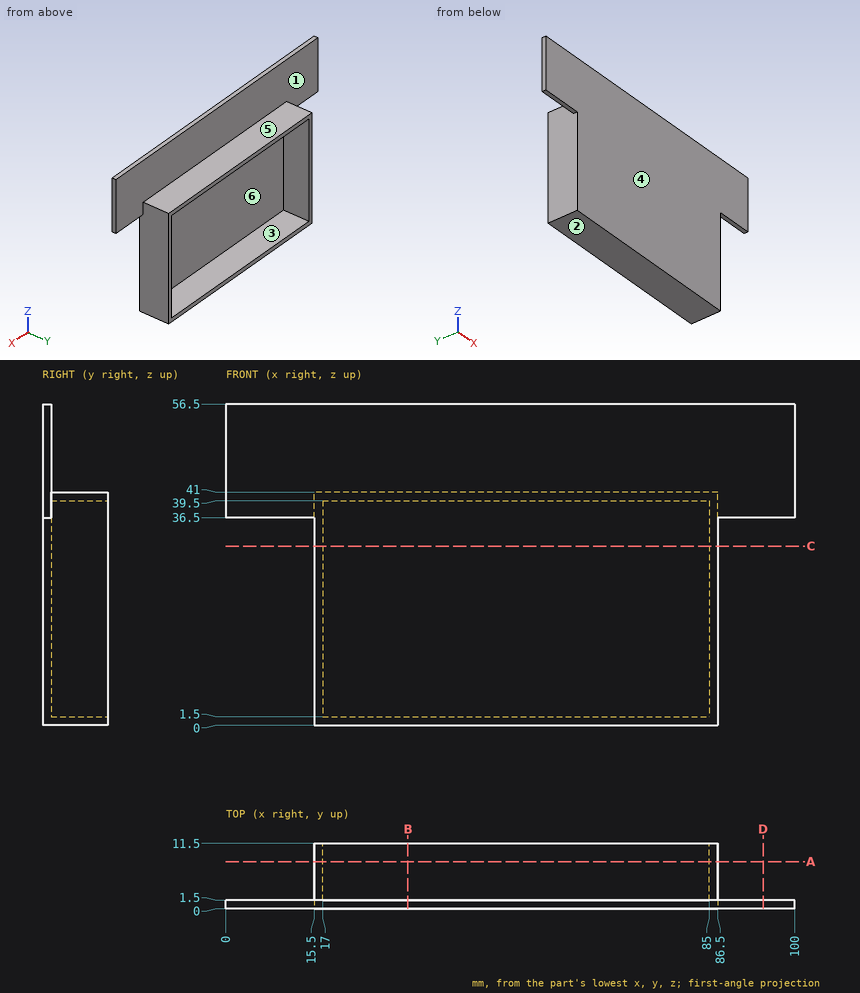
Drawing for the job (mm, zero at the part's lowest x, y, z). A direction names the side the tool comes from. Round coordinates to 2 decimals unless told otherwise and drop trailing zeros. Write each loop counter-clockwise with the first axis right and the second up, starting at its lowest first coordinate (ties: lowest second). Pieces come first, ordered by that corner, then holes. Notation, with made-up numbers: M 23,-18.75 L 49,-18.75 A34 ccw 49,13.25 Z; hole C 9,24 d5. An arc over 180 degrees is marked long. Answer as a JSON object with one key per item and string values. Group by question number.
(1) Cut at B-B (x = 32). Give the cut face in (y, z).
(2) Mould opens along Z. For the marked faces 1, 2 and 3 say: pulls with the +Z half, pulls with the -Z half, needs draft (parallel to the pull), parting line crosses it, or undercut.
(3) Cut at A-A (y = 8.25). Give the cut face in (x, z), and give its area (3 significant figures).
(4) Which spindle directions (+Z, -Z, +X, -X, +Y, -Y) get a long thin tool onto all of the face, cutting with end or side? Do the marked faces 4, 5 and 6. Say none if no direction does.
(5) Flat gauge pins, fed straight in: pin 1 (1.5 mm diameter, centred on y = 7.5, z = 33.5, fed in from -X); pin 2 (6 mm diameter, centred on x = 67.5, z = 48.5, fed in from +Y); pin 3 (3 mm diameter, centred on y = 8.5, z = 33, fed in from +X). Where does each tip first touch, or does it go through?
(6) Cut at C-C (z = 31.5). Give the cut face in (x, y).
(7) Cut at D-D (x = 94.5). Give the cut face in (y, z), and give its area (3 significant figures).
(8) Drill centre lines: L1, parallel to Z at x = 37.5, y = 10.5; L2, parallel to X at y = 1.75, z = 20; L3, parallel to Y at x = 22, z = 15.5. Where is each one in solid material? Low to high.
Responses:
{
 "1": {"outline": "M 0,0 L 11.5,0 L 11.5,1.5 L 1.5,1.5 L 1.5,39.5 L 11.5,39.5 L 11.5,41 L 1.5,41 L 1.5,56.5 L 0,56.5 Z"},
 "2": {"face 1": "needs draft", "face 2": "pulls with the -Z half", "face 3": "undercut"},
 "3": {"outline": "M 15.5,0 L 86.5,0 L 86.5,41 L 15.5,41 Z; hole M 17,1.5 L 85,1.5 L 85,39.5 L 17,39.5 Z", "area": "327 mm2"},
 "4": {"face 4": "+Z, -Z, +X, -X, -Y", "face 5": "+Z, +X, -X, +Y", "face 6": "+Y"},
 "5": {"pin 1": "stops at x = 15.5", "pin 2": "stops at y = 1.5", "pin 3": "stops at x = 86.5"},
 "6": {"outline": "M 15.5,0 L 86.5,0 L 86.5,11.5 L 85,11.5 L 85,1.5 L 17,1.5 L 17,11.5 L 15.5,11.5 Z"},
 "7": {"outline": "M 0,36.5 L 1.5,36.5 L 1.5,56.5 L 0,56.5 Z", "area": "30.0 mm2"},
 "8": {"L1": "z = 0 to 1.5, 39.5 to 41", "L2": "x = 15.5 to 17, 85 to 86.5", "L3": "y = 0 to 1.5"}
}
